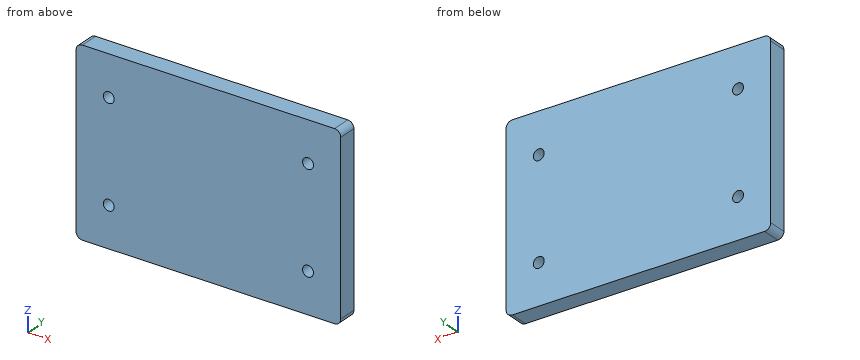
from build123d import *

# Parameters (mm, degrees)
SKETCH_1_W          = 85
SKETCH_1_H          = 58
EXTRUDE_1_DEPTH     = 6
FILLET_1_R          = 2
SKETCH_2_R          = 1.75
CUT_EXTRUDE_1_DEPTH = 6


with BuildPart() as part:
    # 草图1 → 凸台-拉伸1 (new body)
    with BuildSketch(Plane(origin=(0, 0, 0), x_dir=(1, 0, 0), z_dir=(0, 1, 0))):
        Rectangle(SKETCH_1_W, SKETCH_1_H)
    extrude(amount=EXTRUDE_1_DEPTH)

    # 圆角1
    fillet_1_edges = [part.edges().sort_by_distance(p)[0] for p in [
        (42.5, 3, 29),
        (-42.5, 3, 29),
        (-42.5, 3, -29),
        (42.5, 3, -29),
    ]]
    fillet(fillet_1_edges, radius=FILLET_1_R)

    # 草图2 → 切除-拉伸1 (cut)
    with BuildSketch(Plane(origin=(0, 6, 0), x_dir=(1, 0, 0), z_dir=(0, 1, 0))):
        with Locations(Location((-32, 16, 0), (0, 0, 270))):
            Circle(SKETCH_2_R)
        with Locations(Location((32, 16, 0), (0, 0, 90))):
            Circle(SKETCH_2_R)
        with Locations(Location((32, -16, 0), (0, 0, 270))):
            Circle(SKETCH_2_R)
        with Locations(Location((-32, -16, 0), (0, 0, 90))):
            Circle(SKETCH_2_R)
    extrude(amount=-CUT_EXTRUDE_1_DEPTH, mode=Mode.SUBTRACT)


solid = part.part
The listing builds one solid part. Answer for the finished solid, in the listing's coordinates (mm). Coordinates: 2 decimals unless noted, no trailing zeros. Loops run counter-clockwise (first coordinate to the right, second up) from the corner with the lowest first, then second, coordinate; pieces in that order, holes last.
1) Find section B-B on z = 16. Write down the section's boundary in (x, y), then the cut area to 3 significant figures.
2) A flat-ended cylindrical pin translates along its axis: pin 1 Ø4 at (x, z) = (32, -16) entering from +Y. Find the tip coordinate at first contact, or state that the pin passes through.
3) Find section A-A on x = 32. Write down the section's boundary in (y, z), then the cut area to 3 significant figures.
4) Find the intervals of material crossed by L1, parallel to X at y = 0.7, z = 16; L2, parallel to X at y = 0.6, z = -15, in increasing order.
Values:
1. outline: (-42.5, 0) - (-33.75, 0) - (-33.75, 6) - (-42.5, 6) - close; (-30.25, 0) - (30.25, 0) - (30.25, 6) - (-30.25, 6) - close; (33.75, 0) - (42.5, 0) - (42.5, 6) - (33.75, 6) - close
1. area: 468 mm2
2. pin 1: stops at y = 6
3. outline: (0, -29) - (6, -29) - (6, -17.75) - (0, -17.75) - close; (0, -14.25) - (6, -14.25) - (6, 14.25) - (0, 14.25) - close; (0, 17.75) - (6, 17.75) - (6, 29) - (0, 29) - close
3. area: 306 mm2
4. L1: x = -42.5 to -33.75, -30.25 to 30.25, 33.75 to 42.5
4. L2: x = -42.5 to -33.44, -30.56 to 30.56, 33.44 to 42.5
